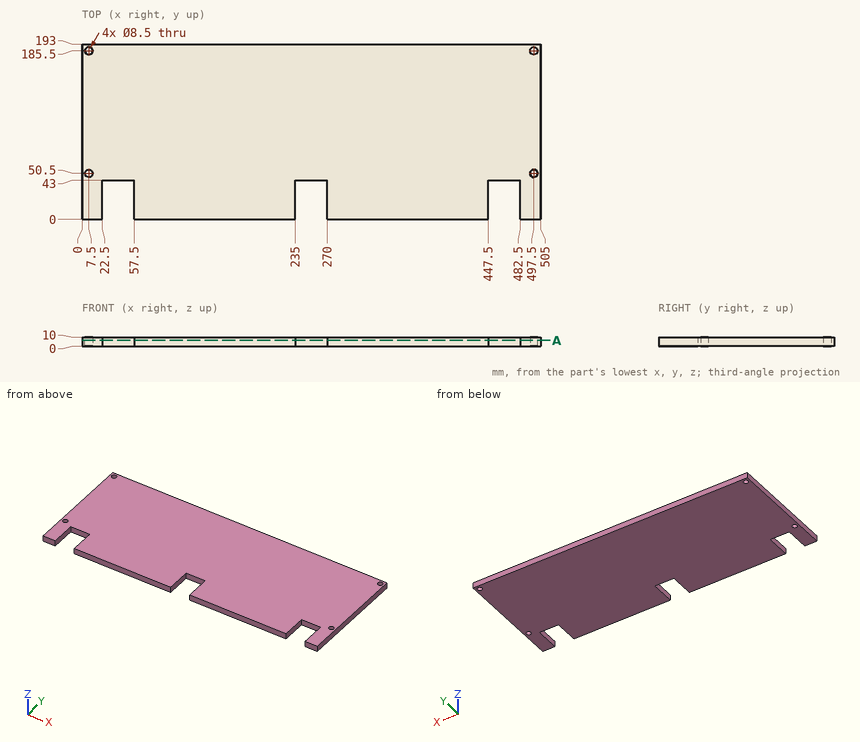
Job drawing, mm, ordinate dimensions from the low corner. One solid piece. Give positions to 0.01 mm unless a question says otherwise; leave off trailing zeros. Write each loop counter-clockwise with the first axis right and the second up, starting at its lowest first coordinate (ties: lowest second). Pieces come first, ordered by that corner, then holes. Notation, with made-up numbers: (82.5, 52) -> (130.5, 52) arc R10 ccw to (130.5, 58) -> close; hole circle Ø3 at (20.25, 5). An arc over 180 degrees is marked (long way). Return JSON: item names as keys, results as strings.
Item 1: Drill centre lines: probe 1 along X at (y, z) = (185.5, 4); probe 2 along Y at (x, z) = (7.5, 6); probe 3 along X at (y, z) = (37, 6.5). Where is each one in solid material? Low to high.
Answer below:
{"probe 1": "x = 0 to 3.25, 11.75 to 493.25, 501.75 to 505", "probe 2": "y = 0 to 46.25, 54.75 to 181.25, 189.75 to 193", "probe 3": "x = 0 to 22.5, 57.5 to 235, 270 to 447.5, 482.5 to 505"}
Item 2: Drop flat-ended pins along their axis: pin 1 (5 mm diameter, centred on x = 31.5, z = 5, fed in from -Y); pin 2 (5 mm diameter, centred on x = 7.5, y = 185.5, fed in from +Z). Give the stop position or say it passes through.
Answer below:
{"pin 1": "stops at y = 43", "pin 2": "passes through"}
Item 3: Band-saw the part on A-A (z = 6.5). List the corners of the cut face in (x, y), then the cut area to 3 significant figures.
Answer below:
{"outline": "(0, 0) -> (22.5, 0) -> (22.5, 43) -> (57.5, 43) -> (57.5, 0) -> (235, 0) -> (235, 43) -> (270, 43) -> (270, 0) -> (447.5, 0) -> (447.5, 43) -> (482.5, 43) -> (482.5, 0) -> (505, 0) -> (505, 193) -> (0, 193) -> close; hole circle Ø8.5 at (7.5, 50.5); hole circle Ø8.5 at (7.5, 185.5); hole circle Ø8.5 at (497.5, 50.5); hole circle Ø8.5 at (497.5, 185.5)", "area": "92,700 mm2"}
